Here's how the part is built. I have some questions about the finished solid (model axes, mm). Round coordinates to 2 decimals unless told otherwise and drop trailing zeros. Order: outer loops, then holes, each group sorted by start corner. A loop starts at its lowest first (then second) coordinate and runs counter-clockwise, first axis right, second up. Notation, with made-up numbers: (25, 71.25) -> (64, 71.25) arc R16 cw to (64, 93.25) -> close; hole circle Ø7 at (-19.5, 44). An arc over 180 degrees is marked (long way). Use a Markdown table: item, result. Add a question column.
(1) I'm going to push a flat-ended pin straight in: P1, Ø4.5, axis at x = 41.25, y = -10.29, coming from the -Z side. Where does the tip first touch, or does it pass through?
(2) I want a section at C-C, the plane x = 33. Please give me the cut outline in (y, z), then the cut area to 3 significant figures.
(3) If I drill on probe 1 along X at (y, z) = (-111.5, 0.9); probe 2 along X at (y, z) = (-63, 1.85); probe 3 along X at (y, z) = (-114, 0.65), over which ranges is the centre line in solid material (lowest first)?
(4) I want a section at A-A, the plane y = -36.5. Please give me the cut outline in (x, z), then the cut area to 3 significant figures.
(5) I want a section at B-B, the plane x = 86.5. Please give me the cut outline in (y, z).
(6) I want a section at D-D, the plane z = 0.6. Give the number of separate pieces and of enclosed holes in the cut face, then the cut area to 3 significant figures.
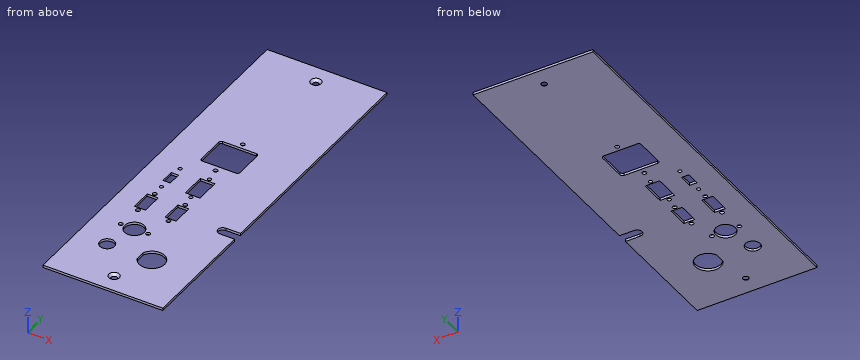
from build123d import *

# Parameters (mm, degrees)
SKIZZE2_W                                   = 98
SKIZZE2_H                                   = 300
AUFSATZ_LINEAR_AUSTRAGEN1_DEPTH             = 2
FORMSENKUNG_F_R_M4_SENKSCHRAUBE_MIT_2_COUNT = 2
FORMSENKUNG_F_R_M4_SENKSCHRAUBE_MIT_2_PITCH = 270
SKIZZE6_R                                   = 1.7
SKIZZE6_R_2                                 = 8
SKIZZE6_R_3                                 = 1.5
SKIZZE6_R_4                                 = 6
SKIZZE6_R_5                                 = 1.75
SKIZZE6_W                                   = 9
SKIZZE6_H                                   = 17
SKIZZE6_W_2                                 = 12
SKIZZE6_H_2                                 = 20
SKIZZE6_W_3                                 = 6
SKIZZE6_H_3                                 = 11
SCHNITT_LINEAR_AUSTRAGEN1_DEPTH             = 10


with BuildPart() as part:
    # Skizze2 → Aufsatz-Linear austragen1 (new body)
    with BuildSketch(Plane.XY):
        with Locations((46, -55.288461538)):
            Rectangle(SKIZZE2_W, SKIZZE2_H)
    extrude(amount=AUFSATZ_LINEAR_AUSTRAGEN1_DEPTH)

    # Skizze4 → Formsenkung für M4 Senkschraube mit Innensechskant1 (revolve, cut)
    with BuildSketch(Plane(origin=(46, 79.711538462, 2), x_dir=(0, -1, 0), z_dir=(1, 0, 0))):
        Polygon((0, 0), (0, 2), (2.25, 2), (2.25, 2.05), (4.3, 0), align=None)
    formsenkung_f_r_m4_senkschraube_mit_inne = revolve(axis=Axis((46, 79.711538462, 8.35), (0, 0, -1)), mode=Mode.SUBTRACT)

    # Formsenkung f_r M4 Senkschraube mit  2: Formsenkung für M4 Senkschraube mit Innensechskant1 ×2
    with Locations(*[(0, -i * FORMSENKUNG_F_R_M4_SENKSCHRAUBE_MIT_2_PITCH, 0) for i in range(1, FORMSENKUNG_F_R_M4_SENKSCHRAUBE_MIT_2_COUNT)]):
        add(formsenkung_f_r_m4_senkschraube_mit_inne, mode=Mode.SUBTRACT)

    # Skizze6 → Schnitt-Linear austragen1 (cut)
    with BuildSketch(Plane.XY.offset(2)):
        with Locations((41.25, -10.288461538)):
            Circle(SKIZZE6_R)
        with Locations((41.25, -46.688461538)):
            Circle(SKIZZE6_R)
        with Locations((44.5, -92.538461538)):
            Circle(SKIZZE6_R)
        with Locations((44.5, -115.038461538)):
            Circle(SKIZZE6_R)
        with Locations((29, -135.288461538)):
            Circle(SKIZZE6_R_2)
        with Locations((43, -57.788461538)):
            Circle(SKIZZE6_R_3)
        with Locations((43, -82.788461538)):
            Circle(SKIZZE6_R_3)
        with Locations((22, -160.288461538)):
            Circle(SKIZZE6_R_4)
        with Locations((40.2, -135.288461538)):
            Circle(SKIZZE6_R_5)
        with Locations((17.8, -135.288461538)):
            Circle(SKIZZE6_R_5)
        with Locations((19.5, -115.038461538)):
            Circle(SKIZZE6_R)
        with Locations((19.5, -92.538461538)):
            Circle(SKIZZE6_R)
        with Locations((19, -57.788461538)):
            Circle(SKIZZE6_R_3)
        with Locations((19, -82.788461538)):
            Circle(SKIZZE6_R_3)
        with BuildLine():
            Line((27.5, -14.688461538), (55, -14.688461538))
            ThreePointArc((55, -14.688461538), (56.414213562, -15.274247976), (57, -16.688461538))
            Line((57, -16.688461538), (57, -39.888461538))
            ThreePointArc((57, -39.888461538), (56.414213562, -41.302675101), (55, -41.888461538))
            Line((55, -41.888461538), (27.5, -41.888461538))
            ThreePointArc((27.5, -41.888461538), (26.085786438, -41.302675101), (25.5, -39.888461538))
            Line((25.5, -39.888461538), (25.5, -16.688461538))
            ThreePointArc((25.5, -16.688461538), (26.085786438, -15.274247976), (27.5, -14.688461538))
        make_face()
        with Locations((44.5, -103.788461538)):
            Rectangle(SKIZZE6_W, SKIZZE6_H)
        with Locations((43, -70.288461538)):
            Rectangle(SKIZZE6_W_2, SKIZZE6_H_2)
        with Locations((19, -70.288461538)):
            Rectangle(SKIZZE6_W_3, SKIZZE6_H_3)
        with BuildLine():
            Line((49, -164.223004079), (49, -156.353918998))
            ThreePointArc((49, -156.353918998), (68.975, -160.288461538), (49, -164.223004079))
        make_face()
        with Locations((19.5, -103.788461538)):
            Rectangle(SKIZZE6_W, SKIZZE6_H)
        with BuildLine():
            Line((95, -101.288461538), (83, -101.288461538))
            ThreePointArc((83, -101.288461538), (79, -105.288461538), (83, -109.288461538))
            Line((83, -109.288461538), (95, -109.288461538))
            Line((95, -109.288461538), (95, -101.288461538))
        make_face()
    extrude(amount=-SCHNITT_LINEAR_AUSTRAGEN1_DEPTH, mode=Mode.SUBTRACT)


solid = part.part
Taken from the geometry:
| question | item | result |
|---|---|---|
| 1 | P1 | stops at z = 0 |
| 2 | outline | (-205.29, 0) -> (-142.22, 0) -> (-142.22, 2) -> (-205.29, 2) -> close; (-128.36, 0) -> (-41.89, 0) -> (-41.89, 2) -> (-128.36, 2) -> close; (-14.69, 0) -> (94.71, 0) -> (94.71, 2) -> (-14.69, 2) -> close |
| 2 | area | 518 mm2 |
| 3 | probe 1 | x = -3 to 15, 24 to 40, 49 to 95 |
| 3 | probe 2 | x = -3 to 37, 49 to 95 |
| 3 | probe 3 | x = -3 to 18.15, 20.85 to 43.15, 45.85 to 95 |
| 4 | outline | (-3, 0) -> (25.5, 0) -> (25.5, 2) -> (-3, 2) -> close; (57, 0) -> (95, 0) -> (95, 2) -> (57, 2) -> close |
| 4 | area | 133 mm2 |
| 5 | outline | (-205.29, 0) -> (-109.29, 0) -> (-109.29, 2) -> (-205.29, 2) -> close; (-101.29, 0) -> (94.71, 0) -> (94.71, 2) -> (-101.29, 2) -> close |
| 6 | separate pieces | 1 |
| 6 | enclosed holes | 22 |
| 6 | area | 27,000 mm2 |
